Job drawing, mm, ordinate dimensions from the low corner. One solid piece. Give positions to 0.01 mm unless a question says otherwise; leave off trailing zeros. Write each loop counter-clockwise with the first axis right and the second up, starting at its lowest first coordinate (ties: lowest second). Pieces come first, ordered by that corner, then holes. Notation, with made-up numbers: M 68.5,-25 L 82.5,-25 A16 cw 82.5,3 Z; hole C 31,5 d4. An arc over 180 degrees is marked long. Answer as CSV lines item,"result". Start each with the question number.
Item 1: Band-saw the part on C-C, the plane z = 5. List the corners of the cut face in (x, y) (1 decimal).
Item 2: Band-saw the part on D-D, the plane y = 4.5. List the corners of the cut face in (x, z) (1 decimal).
Item 3: Two-plate mould, pull along X, no slides. Class the marked faces 1, 2 and 3: +X half, -X half, draft (parallel to the pull), parting line (faces both ways), or undercut.
Item 4: Wall check: L1, parallel to X at y = 20.5, z = 7 (1 decimal); L2, parallel to Y at x = 15.25, z = 4.5 (1 decimal); L3, parallel to X at y = 12, z = 5. Give the ranges that are in metal, low to high. Write a range as from..to.
Item 5: Band-saw the part on B-B, the plane x = 10. List the corners of the cut face in (y, z) (1 decimal), then the cut area to 3 significant figures.
Item 6: Band-saw the part on A-A, the plane y = 18. List the corners of the cut face in (x, z) (1 decimal), then the cut area to 3 significant figures.
Item 7: Pin check, flat tip, straight feed: pin 1 (1.5 mm diameter, centred on x = 4, z = 7.5, fed in from -Y). Stop position of the tip, or through.
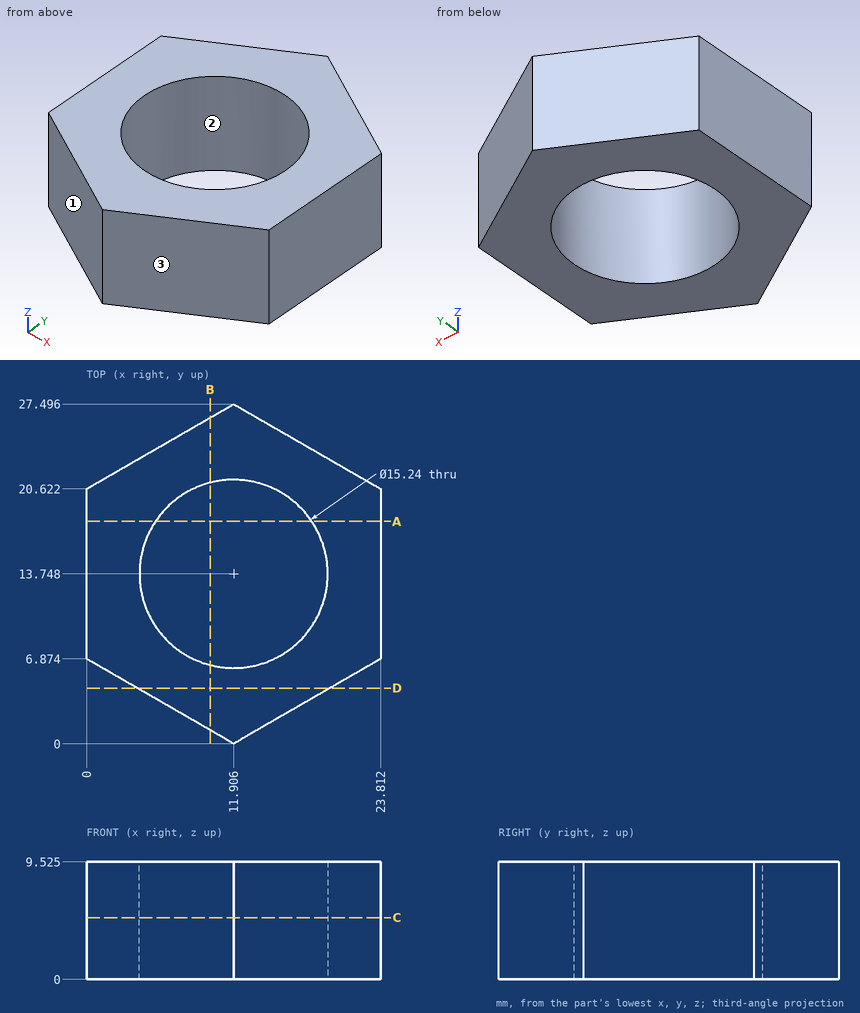
Output:
1,outline,"M 0,6.9 L 11.9,0 L 23.8,6.9 L 23.8,20.6 L 11.9,27.5 L 0,20.6 Z; hole C 11.9,13.7 d15.2"
2,outline,"M 4.1,0 L 19.7,0 L 19.7,9.5 L 4.1,9.5 Z"
3,face 1,"-X half"
3,face 2,"undercut"
3,face 3,"+X half"
4,L1,"0..8.4, 15.4..23.8"
4,L2,"1.9..6.9, 20.6..25.6"
4,L3,"0..4.49, 19.32..23.81"
5,outline,"M 1.1,0 L 6.4,0 L 6.4,9.5 L 1.1,9.5 Z; M 21.1,0 L 26.4,0 L 26.4,9.5 L 21.1,9.5 Z"
5,area,"100 mm²"
6,outline,"M 0,0 L 5.6,0 L 5.6,9.5 L 0,9.5 Z; M 18.2,0 L 23.8,0 L 23.8,9.5 L 18.2,9.5 Z"
6,area,"106 mm²"
7,pin 1,"y = 4.13"
